Source: three-view drawing plus pictorial views. Frame: mm from the lowest corner of the part. Coordinates: 2 decimals unless noted, no trailing zeros. Write each loop counter-clockwise with the first axis right and the second up, starting at its lowest first coordinate (ties: lowest second). Pieces come first, ordered by that corner, then holes. Notation, with made-up numbers: M 19,32.5 L 71,32.5 A5 ccw 71,38.5 Z; hole C 27,89 d9. An arc over 180 degrees is marked long. Write item = value, one per line. Start each with the question number.
Item 1: Section D-D on y = 71. Output: boundary loops of the cut face in (x, z), plus the area to 3 significant figures.
Item 2: Ray query, L1, parallel to Y at x = 0.2, z = 29.5 (1 decimal); L2, parallel to Y at x = 0.35, z = 25.5 (1 decimal); L3, parallel to Y at x = 0.35, z = 14.5 (1 decimal). Return the intervals inside material, ascending. Write a range as [from, to].
Item 3: Section A-A on z = 28. Output: boundary loops of the cut face in (x, y) (1 decimal).
Item 4: Section B-B on z = 22.5. Output: boundary loops of the cut face in (x, y) (1 decimal).
Item 5: First-contact query: pin 1 Ø0.5 at (x, y) = (0.5, 26.5) entering from +Z; pin 2 Ø0.5 at (x, y) = (0.5, 46) entering from +Z. Flat tips, straight axial feed; report the tip coordinate or a pass-through.
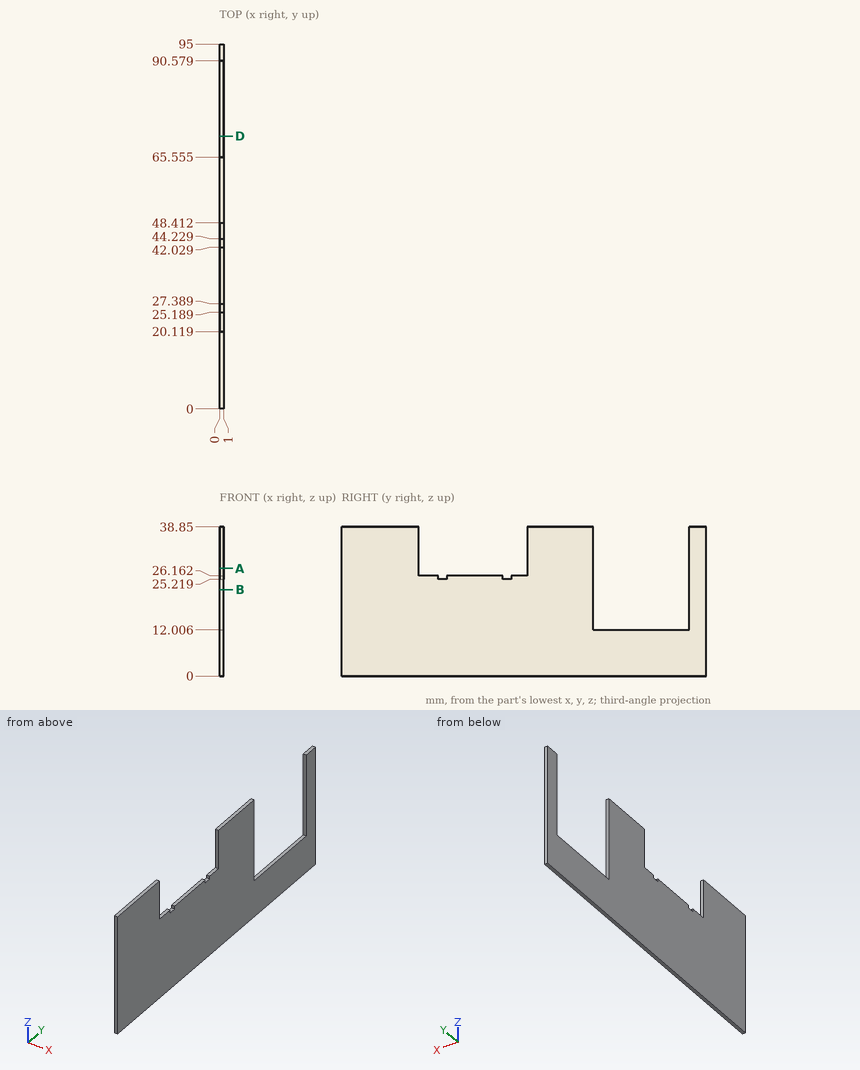
Responses:
q1.outline = M 0,0 L 1,0 L 1,12.01 L 0,12.01 Z
q1.area = 12.0 mm²
q2.L1 = [0, 20.1], [48.4, 65.6], [90.6, 95]
q2.L2 = [0, 25.2], [27.4, 42], [44.2, 65.6], [90.6, 95]
q2.L3 = [0, 65.6], [90.6, 95]
q3.outline = M 0,0 L 1,0 L 1,20.1 L 0,20.1 Z; M 0,48.4 L 1,48.4 L 1,65.6 L 0,65.6 Z; M 0,90.6 L 1,90.6 L 1,95 L 0,95 Z
q4.outline = M 0,0 L 1,0 L 1,65.6 L 0,65.6 Z; M 0,90.6 L 1,90.6 L 1,95 L 0,95 Z
q5.pin_1 = 25.22
q5.pin_2 = 26.16
